The model under review builds one solid part; all positions refer to its coordinate system, in mm. Coordinates: 2 decimals unless noted, no trailing zeros. Loops run counter-clockwise (first coordinate to the right, second up) from the corner with the lowest first, then second, coordinate; pieces in that order, holes last. Notation, with made-up numbers: (40.25, -0.5) - (81.25, -0.5) arc R31 cw to (81.25, 25.5) - close; hole circle Ø9 at (29, 10). An arc over 180 degrees is marked (long way). One line per item, written item: value. Start each with the question number.
1. We need section D-D, the plane x = 13. Give the boundary of the cut face in (y, z).
2. To check wall thickness, follow line 1 (X direction, y = 8, z = 1.55); line 2 (X direction, y = -6, z = 1.6); line 3 (Y direction, x = -13, z = 1.05). State the ranges of each line that lie inside material, in increasing order.
3. We need section C-C, the plane x = -12.7. Give the boundary of the cut face in (y, z), then the cut area to 3 significant figures.
4. We need section A-A, the plane y = 18. Give the boundary of the cut face in (x, z).
5. We need section B-B, the plane z = 1.7. Give the boundary of the cut face in (x, y).
from build123d import *

# Parameters (mm, degrees)
SKETCH_1_W          = 35
SKETCH_1_H          = 55
EXTRUDE_1_DEPTH     = 2
CUT_EXTRUDE_1_DEPTH = 10
FILLET_1_R          = 2


with BuildPart() as part:
    # Sketch 1 → 凸台-拉伸1 (new body)
    with BuildSketch(Plane.XY):
        Rectangle(SKETCH_1_W, SKETCH_1_H)
    extrude(amount=EXTRUDE_1_DEPTH)

    # 草图9 → 切除-拉伸1 (cut)
    with BuildSketch(Plane.XY.offset(2)):
        with BuildLine():
            Line((14.95, 21.5), (14.95, -4.5))
            ThreePointArc((14.95, -4.5), (12.7, -6.75), (10.45, -4.5))
            Line((10.45, -4.5), (10.45, 21.5))
            ThreePointArc((10.45, 21.5), (12.7, 23.75), (14.95, 21.5))
        make_face()
        with BuildLine():
            Line((-14.95, 21.5), (-14.95, -4.5))
            ThreePointArc((-14.95, -4.5), (-12.7, -6.75), (-10.45, -4.5))
            Line((-10.45, -4.5), (-10.45, 21.5))
            ThreePointArc((-10.45, 21.5), (-12.7, 23.75), (-14.95, 21.5))
        make_face()
    extrude(amount=-CUT_EXTRUDE_1_DEPTH, mode=Mode.SUBTRACT)

    # 圆角1
    fillet_1_edges = [part.edges().sort_by_distance(p)[0] for p in [
        (17.5, 27.5, 1),
        (17.5, -27.5, 1),
        (-17.5, -27.5, 1),
        (-17.5, 27.5, 1),
    ]]
    fillet(fillet_1_edges, radius=FILLET_1_R)


solid = part.part
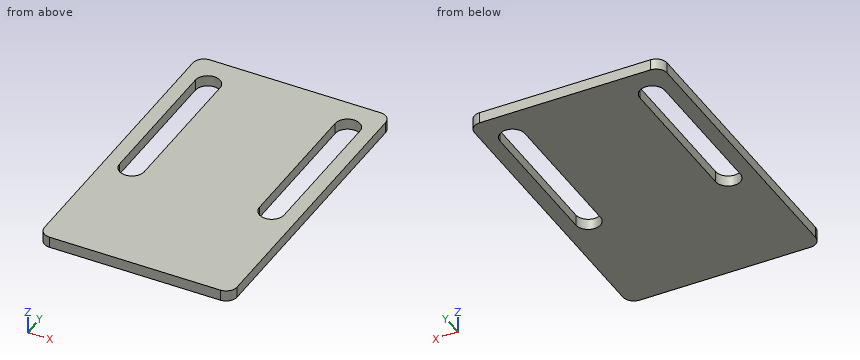
Findings below:
1. outline: (-27.5, 0) - (-6.73, 0) - (-6.73, 2) - (-27.5, 2) - close; (23.73, 0) - (27.5, 0) - (27.5, 2) - (23.73, 2) - close
2. line 1: -17.5 to -14.95, -10.45 to 10.45, 14.95 to 17.5
2. line 2: -17.5 to -14.38, -11.02 to 11.02, 14.38 to 17.5
2. line 3: -27.5 to -6.73, 23.73 to 27.5
3. outline: (-27.5, 0) - (-6.75, 0) - (-6.75, 2) - (-27.5, 2) - close; (23.75, 0) - (27.5, 0) - (27.5, 2) - (23.75, 2) - close
3. area: 49.0 mm2
4. outline: (-17.5, 0) - (-14.95, 0) - (-14.95, 2) - (-17.5, 2) - close; (-10.45, 0) - (10.45, 0) - (10.45, 2) - (-10.45, 2) - close; (14.95, 0) - (17.5, 0) - (17.5, 2) - (14.95, 2) - close
5. outline: (-17.5, -25.5) arc R2 ccw to (-15.5, -27.5) - (15.5, -27.5) arc R2 ccw to (17.5, -25.5) - (17.5, 25.5) arc R2 ccw to (15.5, 27.5) - (-15.5, 27.5) arc R2 ccw to (-17.5, 25.5) - close; hole (-14.95, -4.5) arc R2.25 ccw to (-10.45, -4.5) - (-10.45, 21.5) arc R2.25 ccw to (-14.95, 21.5) - close; hole (10.45, -4.5) arc R2.25 ccw to (14.95, -4.5) - (14.95, 21.5) arc R2.25 ccw to (10.45, 21.5) - close
